Input: dimensioned drawing with shaded views. Units: mm. Origin: part minimum x, y, z. A direction names the side the tool comes from. Round coordinates to 2 decimals unless told otherwise and drop trailing zeros. Write each loop counter-clockwise with the first axis right and the second up, starting at its lowest first coordinate (ties: lowest second). Pieces come first, ordered by that corner, then holes. Notation, with made-up numbers: M 87,13.25 L 137,13.25 A18 ccw 137,17.25 Z; hole C -13,57 d5. An arc over 180 degrees is marked long. Put each result on its own line as item: value. Start each with the question number.
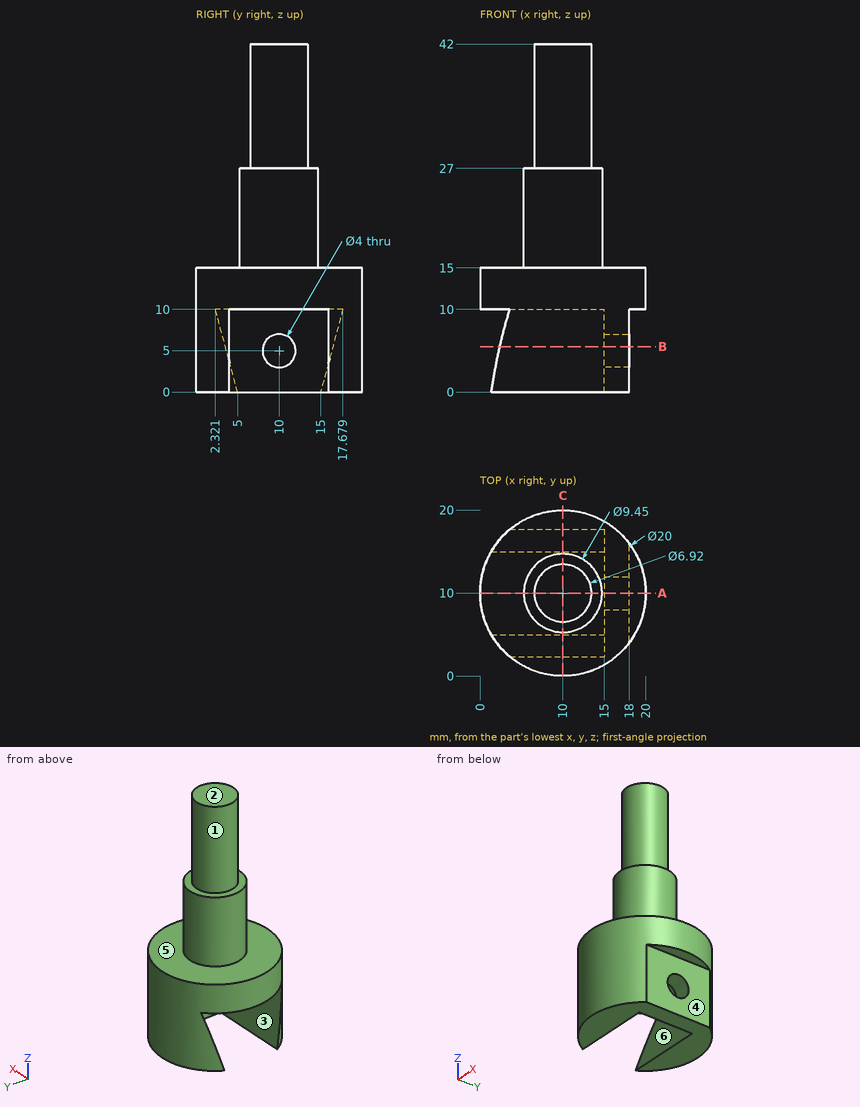
1) Access query for the marked faces 4, 5 and 6. Directions: +Z, -Z, +X, -X, +Y, -Y. A direction counts if a zero-diameter tool reaches every point of the face in a straight line with its end or side. Return the directions, or none.
2) Draft query along Y for the marked faces 1, 2 and 3. Return one class per face: +Y half, -Y half, draft (parallel to the pull), parting line (faces both ways), or undercut.
3) Section B-B, the plane z = 5.5. Output: boundary loops of the cut face in (x, y).
4) First-contact query: pin 1 (8 mm diameter, centred on y = 10.5, z = 3.5, fed in from +X); pin 2 (1 mm diameter, centred on y = 9, z = 14, fed in from -X); pin 3 (8 mm diameter, centred on y = 12.5, z = 34, fed in from -X). Flat tips, straight axial feed; report the tip coordinate or a pass-through.
5) Ray query, probe 1 along Z at (x, y) = (2.5, 9.75); probe 2 along Z at (x, y) = (11.5, 11); probe 3 along Y at (x, z) = (15.85, 5). Return the intervals inside material, ascending.
6) Section A-A, the plane y = 10. Output: boundary loops of the cut face in (x, z) (1 decimal).
7) Section C-C, the plane x = 10. Output: boundary loops of the cut face in (y, z) (1 decimal).
Solved:
1. face 4: -Z, +X, +Y, -Y
1. face 5: +Z
1. face 6: -X
2. face 1: parting line
2. face 2: draft
2. face 3: undercut
3. outline: M 2.38,3.53 A10 ccw 18,4 L 18,8.06 L 15,8.06 L 15,3.53 Z; M 2.38,16.47 L 15,16.47 L 15,11.94 L 18,11.94 L 18,16 A10 ccw Z
4. pin 1: stops at x = 18
4. pin 2: stops at x = 0.01
4. pin 3: stops at x = 6.54
5. probe 1: z = 10 to 15
5. probe 2: z = 10 to 42
5. probe 3: y = 1.89 to 8, 12 to 18.11
6. outline: M 0,10 L 15,10 L 15,7 L 18,7 L 18,10 L 20,10 L 20,15 L 14.7,15 L 14.7,27 L 13.5,27 L 13.5,42 L 6.5,42 L 6.5,27 L 5.3,27 L 5.3,15 L 0,15 Z; M 15,0 L 18,0 L 18,3 L 15,3 Z
7. outline: M 0,0 L 5,0 L 2.3,10 L 17.7,10 L 15,0 L 20,0 L 20,15 L 14.7,15 L 14.7,27 L 13.5,27 L 13.5,42 L 6.5,42 L 6.5,27 L 5.3,27 L 5.3,15 L 0,15 Z
